from build123d import *

# Parameters (mm, degrees)
F0_R     = 4.25
F0_R_2   = 64.727352
F0_R_3   = 35
F0_R_4   = 25
F1_DEPTH = 25
F2_DEPTH = 5
F0_R_5   = 5
F3_DEPTH = 10
F4_R     = 2


with BuildPart() as f1:
    # F0 (on Front) → F1 (new body)
    with BuildSketch(Plane.XZ):
        with BuildLine():
            Line((-79.221434, 8.551697), (-79.221434, -62.172039))
            ThreePointArc((-79.221434, -62.172039), (-73.337461, -76.340236), (-59.147655, -82.171903))
            Line((-59.147655, -82.171903), (122.501798, -81.501799))
            Line((122.501798, -81.501799), (171.501798, -81.501799))
            ThreePointArc((171.501798, -81.501799), (211.272403, -37.224069), (162.995402, -2.416748))
            ThreePointArc((162.995402, -2.416748), (142.222809, 19.4504), (150.953003, 48.320045))
            Line((150.953003, 48.320045), (191.960681, 86.556595))
            ThreePointArc((191.960681, 86.556595), (197.380732, 123.673205), (162.342815, 137.065893))
            Line((162.342815, 137.065893), (-30.592394, 75.209645))
            ThreePointArc((-30.592394, 75.209645), (-65.772151, 49.807198), (-79.221434, 8.551697))
        make_face()
        with Locations((-59.221434, -62.172039)):
            Circle(F0_R, mode=Mode.SUBTRACT)
        with Locations((-9.221434, 8.551697)):
            Circle(F0_R_2, mode=Mode.SUBTRACT)
        with BuildLine():
            ThreePointArc((-39.281463, -63.720447), (-36.417231, -58.822506), (-30.797483, -58.040151))
            ThreePointArc((-30.797483, -58.040151), (56.444701, -15.696162), (17.658669, 73.184971))
            ThreePointArc((17.658669, 73.184971), (13.660211, 79.454771), (18.161905, 85.373623))
            Line((18.161905, 85.373623), (133.888191, 122.647992))
            ThreePointArc((133.888191, 122.647992), (140.261736, 121.262963), (142.2244, 115.042968))
            ThreePointArc((142.2244, 115.042968), (145.633078, 93.30579), (162.956944, 79.740846))
            ThreePointArc((162.956944, 79.740846), (167.433191, 74.997051), (165.538317, 68.756071))
            Line((165.538317, 68.756071), (147.543189, 51.97698))
            ThreePointArc((147.543189, 51.97698), (136.412702, 26.139516), (147.894897, 0.456418))
            ThreePointArc((147.894897, 0.456418), (150.020686, -4.654258), (147.437848, -9.549861))
            ThreePointArc((147.437848, -9.549861), (137.009777, -21.245923), (131.874992, -36.050534))
            ThreePointArc((131.874992, -36.050534), (129.428981, -40.293368), (124.716016, -41.624746))
            ThreePointArc((124.716016, -41.624746), (106.920259, -48.963232), (103.558552, -67.916893))
            ThreePointArc((103.558552, -67.916893), (102.684131, -73.789814), (97.401997, -76.501799))
            Line((97.401997, -76.501799), (-33.904545, -76.501799))
            ThreePointArc((-33.904545, -76.501799), (-39.135859, -73.859694), (-40.114348, -68.081292))
            ThreePointArc((-40.114348, -68.081292), (-39.576526, -65.924052), (-39.281463, -63.720447))
        make_face(mode=Mode.SUBTRACT)
        with Locations((122.501798, -61.501799)):
            Circle(F0_R, mode=Mode.SUBTRACT)
        with Locations((171.501798, -41.501799)):
            Circle(F0_R_3, mode=Mode.SUBTRACT)
        with Locations((171.501798, 108.498201)):
            Circle(F0_R_4, mode=Mode.SUBTRACT)
    extrude(amount=F1_DEPTH)

    # F0 (on Front) → F2 (join)
    with BuildSketch(Plane.XZ):
        with BuildLine():
            ThreePointArc((17.658669, 73.184971), (56.444701, -15.696162), (-30.797483, -58.040151))
            ThreePointArc((-30.797483, -58.040151), (-36.417231, -58.822506), (-39.281463, -63.720447))
            ThreePointArc((-39.281463, -63.720447), (-39.576526, -65.924052), (-40.114348, -68.081292))
            ThreePointArc((-40.114348, -68.081292), (-39.135859, -73.859694), (-33.904545, -76.501799))
            Line((-33.904545, -76.501799), (97.401997, -76.501799))
            ThreePointArc((97.401997, -76.501799), (102.684131, -73.789814), (103.558552, -67.916893))
            ThreePointArc((103.558552, -67.916893), (106.920259, -48.963232), (124.716016, -41.624746))
            ThreePointArc((124.716016, -41.624746), (129.428981, -40.293368), (131.874992, -36.050534))
            ThreePointArc((131.874992, -36.050534), (137.009777, -21.245923), (147.437848, -9.549861))
            ThreePointArc((147.437848, -9.549861), (150.020686, -4.654258), (147.894897, 0.456418))
            ThreePointArc((147.894897, 0.456418), (136.412702, 26.139516), (147.543189, 51.97698))
            Line((147.543189, 51.97698), (165.538317, 68.756071))
            ThreePointArc((165.538317, 68.756071), (167.433191, 74.997051), (162.956944, 79.740846))
            ThreePointArc((162.956944, 79.740846), (145.633078, 93.30579), (142.2244, 115.042968))
            ThreePointArc((142.2244, 115.042968), (140.261736, 121.262963), (133.888191, 122.647992))
            Line((133.888191, 122.647992), (18.161905, 85.373623))
            ThreePointArc((18.161905, 85.373623), (13.660211, 79.454771), (17.658669, 73.184971))
        make_face()
    extrude(amount=F2_DEPTH)

    # F0 (on Front) → F3 (join)
    with BuildSketch(Plane.XZ):
        with Locations((-9.221434, 8.551697)):
            Circle(F0_R_2)
        with BuildLine():
            ThreePointArc((-63.940752, -1.277816), (-59.884955, 4.514463), (-54.092675, 0.458665))
            ThreePointArc((-54.092675, 0.458665), (-41.235719, -24.239316), (-16.537738, -37.096272))
            ThreePointArc((-16.537738, -37.096272), (-12.48194, -42.888551), (-18.27422, -46.944349))
            ThreePointArc((-18.27422, -46.944349), (-48.306787, -31.310384), (-63.940752, -1.277816))
        make_face(mode=Mode.SUBTRACT)
        with Locations((-27.634205, -23.340158)):
            Circle(F0_R_5, mode=Mode.SUBTRACT)
        with Locations((-46.046976, 8.551697)):
            Circle(F0_R_5, mode=Mode.SUBTRACT)
        with Locations((9.191337, -23.340158)):
            Circle(F0_R_5, mode=Mode.SUBTRACT)
        with BuildLine():
            ThreePointArc((46.944348, -1.277816), (31.310383, -31.310384), (1.277815, -46.944349))
            ThreePointArc((1.277815, -46.944349), (-4.514464, -42.888551), (-0.458666, -37.096272))
            ThreePointArc((-0.458666, -37.096272), (24.239315, -24.239316), (37.096271, 0.458665))
            ThreePointArc((37.096271, 0.458665), (42.88855, 4.514463), (46.944348, -1.277816))
        make_face(mode=Mode.SUBTRACT)
        with Locations((27.604108, 8.551697)):
            Circle(F0_R_5, mode=Mode.SUBTRACT)
        with BuildLine():
            ThreePointArc((-63.940752, 18.274219), (-48.306787, 48.306786), (-18.27422, 63.940752))
            ThreePointArc((-18.27422, 63.940752), (-12.48194, 59.884954), (-16.537738, 54.092674))
            ThreePointArc((-16.537738, 54.092674), (-41.235719, 41.235719), (-54.092675, 16.537737))
            ThreePointArc((-54.092675, 16.537737), (-59.884955, 12.481939), (-63.940752, 18.274219))
        make_face(mode=Mode.SUBTRACT)
        with Locations((-27.634205, 40.443552)):
            Circle(F0_R_5, mode=Mode.SUBTRACT)
        with Locations((9.191337, 40.443552)):
            Circle(F0_R_5, mode=Mode.SUBTRACT)
        with BuildLine():
            ThreePointArc((46.221116, 18.327714), (42.165318, 12.535435), (36.373039, 16.591232))
            ThreePointArc((36.373039, 16.591232), (23.516083, 41.289214), (-1.181898, 54.14617))
            ThreePointArc((-1.181898, 54.14617), (-5.237696, 59.938449), (0.554583, 63.994247))
            ThreePointArc((0.554583, 63.994247), (30.587151, 48.360282), (46.221116, 18.327714))
        make_face(mode=Mode.SUBTRACT)
    extrude(amount=F3_DEPTH)

    # F4
    f4_edges = [f1.edges().sort_by_distance(p)[0] for p in [
        (13.660211, -5, 79.454771),
        (56.444701, -5, -15.696162),
        (-36.417231, -5, -58.822506),
        (-39.576526, -5, -65.924052),
        (-39.135859, -5, -73.859694),
        (31.748726, -5, -76.501799),
        (102.684131, -5, -73.789814),
        (106.920259, -5, -48.963232),
        (129.428981, -5, -40.293368),
        (137.009777, -5, -21.245923),
        (150.020686, -5, -4.654258),
        (136.412702, -5, 26.139516),
        (156.540753, -5, 60.366526),
        (167.433191, -5, 74.997051),
        (145.633078, -5, 93.30579),
        (140.261736, -5, 121.262963),
        (76.025048, -5, 104.010807),
    ]]
    fillet(f4_edges, radius=F4_R)


solid = f1.part
Read the model definition and answer for the solid it produces. Units are mm, in the model's axes. A direction names the side the tool comes from. Round coordinates to 2 decimals unless told otherwise and drop trailing zeros. Use a Markdown table: item, result.
(1) Straight lines are drawn through the part: line 1 along Z through (x, y) = (-29.5, -4.75); line 2 along X through (y, z) = (-21.75, -71); line 3 along X through (y, z) = (-15.25, -19.5). For each, find the intervals that lie inside material, in ascending order. Write a range as [from, to].
Reported:
| item | result |
|---|---|
| line 1 | [-82.06, -43.74], [-32.76, -27.98], [-18.7, 35.8], [45.08, 49.76], [60.73, 75.56] |
| line 2 | [-77.17, -40.33], [103.82, 152.66], [190.34, 198.52] |
| line 3 | [-79.22, -67.55], [49.11, 54.91], [138.1, 144.28], [198.72, 204.91] |
(2) The mould has two halves that part along X. Classify faces 1 (the flat face through (147, -12, -81.502)), 2 (the flat face through (171.2, -12.3, 67.2)), 3 (the flat face through (-10, -10, 9)): released by +X, released by -X, zero draft, split by the parting line, or undercut.
Reported:
| item | result |
|---|---|
| face 1 | zero draft |
| face 2 | released by +X |
| face 3 | undercut |
(3) The part is cut by section A-A (y = -20.5). State how many separate pieces and enclosed holes the cut face has, then the cut area to 3 significant figures.
Reported:
| item | result |
|---|---|
| separate pieces | 1 |
| enclosed holes | 6 |
| area | 9,700 mm2 |
(4) Each of these flat-tipped pins is pushed along its axis until it touches: pin 1 Ø12 at (x, y) = (42, -12) entering from +Z; pin 2 Ø8 at (x, z) = (103, 105.5) entering from -Y; pin 3 Ø14.5 at (x, y) = (46.5, -14.5) entering from +Z. Where does it stop, or does it pass through?
Reported:
| item | result |
|---|---|
| pin 1 | z = 100.41 |
| pin 2 | y = -5 |
| pin 3 | z = 102.25 |
(5) Which of the six approach directions +Z, -Z, +X, -X, +Y, -Y give full straight-line access (tool end or side, diameter ignored) to faces 4 (the cylindrical face through (107.098, -15.874, -48.745)), 5 (the cylindrical face through (31.65, -4.93, -30.97)), 6 (the cylindrical face through (-65.41, -12.32, 50.3))?
Reported:
| item | result |
|---|---|
| face 4 | -Y |
| face 5 | +Y, -Y |
| face 6 | +Z, -X, +Y, -Y |
